Can you work these out from the model? Positions are in its coordinate system, mm. Face numbers are marked on the shaded views. A direction names the side the tool comes from. Round coordinates to 2 decimals unless told otherwise and drop trailing zeros. Write each loop counter-clockwise with the first axis right and the second up, starting at its lowest first coordinate (ties: lowest second). Pieces come first, ordered by that corner, then holes. Notation, with made-up numbers: (-9, 68.5) -> (0, 68.5) arc R16 cw to (0, 78.5) -> close; hole circle Ø6 at (46.25, 86). An arc over 180 degrees is marked (long way). Write item = value, one per line. Start each with the question number.
1) Thinking about a two-plate mould opening in Y: for the marked faces 6, 7 and 8, which applies, +Y half, -Y half, draft (parallel to the pull), parting line (faces both ways), or undercut?
2) Imagine slicing it at D-D, the plane x = 122.5. Please give me the cut outline in (y, z) (3 decimals).
3) If I drill on line 1 (Y direction, x = 51, z = 7.5); line 2 (Y direction, x = 94, z = 2.75); line 3 (Y direction, x = 122.5, z = 11.25), over which ranges is the centre line in solid material (lowest first)?
4) For the marked faces 1, 2, 3, 4 and 5, which set-ups out of +Z, -Z, +X, -X, +Y, -Y let a thin tool reach every point of the face, with its end or its side?
5) I'm going to push flat-ended pins straight in: pin 1 (6 mm diameter, centred on y = 17.5, z = 7, fed in from +X); pin 2 (8 mm diameter, centred on y = 34.5, z = 8, fed in from +X); pin 3 (5 mm diameter, centred on x = 109, z = 11, fed in from +Y). Where does each tip first touch, or does it pass through?
6) Imagine slicing it at C-C, the plane x = 88.5. Please give me the cut outline in (y, z) (3 decimals).
7) Imagine slicing it at B-B, the plane z = 9.5. Please give me the cut outline in (x, y), then the cut area to 3 significant figures.
8) Imagine slicing it at A-A, the plane y = 9. Please give me the cut outline in (x, z) (3 decimals), then the cut area to 3 significant figures.
Autodesk Inventor part; units mm, degrees
ref_plane "YZ Plane" through (0, 0, 0) normal (1, 0, 0) x (0, 1, 0)
ref_plane "XZ Plane" through (0, 0, 0) normal (0, 1, 0) x (-1, 0, 0)
ref_plane "XY Plane" through (0, 0, 0) normal (0, 0, 1) x (1, 0, 0)
sketch "Sketch1" plane through (0, 0, 0) normal (0, 0, 1) x (1, 0, 0)
  line L0 (25.4, 0) -> (0, 38.1)
  line L1 (63.5, 0) -> (25.4, 0)
  line L2 (63.5, 0) -> (63.5, 12.7)
  line L3 (63.5, 12.7) -> (101.6, 12.7)
  line L4 (101.6, 12.7) -> (101.6, 0)
  line L5 (50.8, 25.4) -> (50.8, 50.8)
  line L6 (50.8, 50.8) -> (114.3, 50.8)
  line L7 (114.3, 50.8) -> (114.3, 25.4)
  line L8 (114.3, 25.4) -> (50.8, 25.4)
  line L9 (101.6, 0) -> (152.4, 0)
  line L10 (152.4, 0) -> (127, 76.2)
  line L11 (127, 76.2) -> (101.6, 76.2)
  line L12 (101.6, 76.2) -> (101.6, 101.6)
  line L13 (101.6, 101.6) -> (38.1, 101.6)
  line L14 (38.1, 101.6) -> (38.1, 63.5)
  line L15 (38.1, 63.5) -> (0, 38.1)
  point P0 (0, 0)
extrude "Extrusion1" add sketch "Sketch1" along normal blind 15.875
properties part number "P2-2"
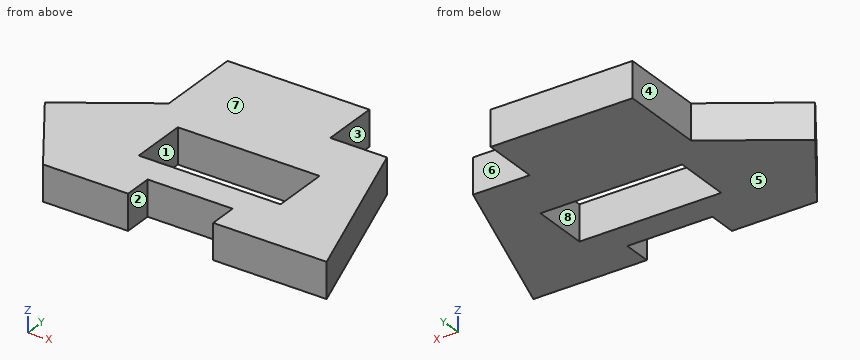
Reported:
q1.face_6 = +Y half
q1.face_7 = draft
q1.face_8 = undercut
q2.outline = (0, 0) -> (76.2, 0) -> (76.2, 15.875) -> (0, 15.875) -> close
q3.line_1 = 0 to 25.4, 50.8 to 101.6
q3.line_2 = 12.7 to 25.4, 50.8 to 101.6
q3.line_3 = 0 to 76.2
q4.face_1 = +Z, -Z
q4.face_2 = +Z, -Z, -Y
q4.face_3 = +Z, -Z, +X, +Y
q4.face_4 = +Z, -Z, -X, +Y
q4.face_5 = -Z, +X, -X, +Y, -Y
q5.pin_1 = 147.57
q5.pin_2 = 142.23
q5.pin_3 = 76.2
q6.outline = (12.7, 0) -> (25.4, 0) -> (25.4, 15.875) -> (12.7, 15.875) -> close; (50.8, 0) -> (101.6, 0) -> (101.6, 15.875) -> (50.8, 15.875) -> close
q7.outline = (0, 38.1) -> (25.4, 0) -> (63.5, 0) -> (63.5, 12.7) -> (101.6, 12.7) -> (101.6, 0) -> (152.4, 0) -> (127, 76.2) -> (101.6, 76.2) -> (101.6, 101.6) -> (38.1, 101.6) -> (38.1, 63.5) -> close; hole (50.8, 25.4) -> (114.3, 25.4) -> (114.3, 50.8) -> (50.8, 50.8) -> close
q7.area = 8,710 mm²
q8.outline = (19.4, 0) -> (63.5, 0) -> (63.5, 15.875) -> (19.4, 15.875) -> close; (101.6, 0) -> (149.4, 0) -> (149.4, 15.875) -> (101.6, 15.875) -> close
q8.area = 1,460 mm²
